Read the model definition and answer for the solid it produces. Units are mm, in the model's axes. A direction names the side the tool comes from. Round coordinates to 2 decimals unless told otherwise and drop trailing zeros. Write each loop counter-clockwise with the first axis right and the second up, starting at its lowest first coordinate (ties: lowest second). Pieces come first, ordered by that corner, then holes.
from build123d import *

# Parameters (mm, degrees)
F0_W     = 145
F0_H     = 185
F1_DEPTH = 55
F3_DEPTH = 98
F5_W     = 120
F5_H     = 28
F6_DEPTH = 25
F7_R     = 5


with BuildPart() as f1:
    # F0 (on Top) → F1 (new body)
    with BuildSketch(Plane.XY):
        Rectangle(F0_W, F0_H)
    extrude(amount=F1_DEPTH)

    # F2 (on Front) → F3 (cut, symmetric)
    with BuildSketch(Plane.XZ):
        Polygon((-92.57464, 55.003494), (-92.79651, 32.817475), (26.113287, 32.817475), (47.771066, 55.003494), align=None)
    extrude(amount=F3_DEPTH, both=True, mode=Mode.SUBTRACT)

    # F5 (on face) → F6 (cut)
    with BuildSketch(Plane.YZ.offset(72.5)):
        with Locations((0.170817, 26)):
            Rectangle(F5_W, F5_H)
    extrude(amount=-F6_DEPTH, mode=Mode.SUBTRACT)

    # F7
    f7_edges = [f1.edges().sort_by_distance(p)[0] for p in [
        (-23.193357, -92.5, 32.817475),
        (36.940471, -92.5, 43.908738),
        (-72.5, 0, 32.817475),
        (-23.193357, 92.5, 32.817475),
        (36.940471, 92.5, 43.908738),
        (47.767656, 0, 55),
        (72.5, 0, 55),
        (60.133828, -92.5, 55),
        (72.5, -92.5, 27.5),
        (72.5, 92.5, 27.5),
        (60.133828, 92.5, 55),
        (0, -92.5, 0),
        (0, 92.5, 0),
        (-72.5, 0, 0),
        (-72.5, -92.5, 16.408738),
        (-72.5, 92.5, 16.408738),
    ]]
    fillet(f7_edges, radius=F7_R)


solid = f1.part
Q1. Section C-C (z = 18) is taken. Determine the outline of the cut face in (x, y), then the cut area to 3 significant figures.
Verdict:
outline: (-72.5, -87.5) arc R5 ccw to (-67.5, -92.5) - (67.5, -92.5) arc R5 ccw to (72.5, -87.5) - (72.5, -59.83) - (47.5, -59.83) - (47.5, 60.17) - (72.5, 60.17) - (72.5, 87.5) arc R5 ccw to (67.5, 92.5) - (-67.5, 92.5) arc R5 ccw to (-72.5, 87.5) - close
area: 23,800 mm2
Q2. Which of the six approach directions +Z, -Z, +X, -X, +Y, -Y give full straight-line access (tool end or side, diameter ignored) to faces 5 (the cylindrical face through (-20.31, -91, 31.39)), 6 (the cylindrical face through (-20.31, 91.074, 31.314)), 7 (the flat face through (60, -1, 40))?
Verdict:
face 5: +Z, -X, -Y
face 6: +Z, -X, +Y
face 7: +X
Q3. Flat-ended cylindrical pins translate along their axes: pin 1 Ø3 at (x, y) = (-46.5, -45) entering from +Z; pin 2 Ø3 at (y, z) = (-39, 49) entering from -X; pin 3 Ø8.5 at (y, z) = (-8.5, 28.5) entering from +X. Find the tip coordinate at first contact, or state that the pin passes through.
Verdict:
pin 1: stops at z = 32.82
pin 2: stops at x = 40.45
pin 3: stops at x = 47.5
Q4. Section A-A (y = 56) is taken. Determine the outline of the cut face in (x, z), then the cut area to 3 significant figures.
Verdict:
outline: (-72.5, 5) arc R5 ccw to (-67.5, 0) - (72.5, 0) - (72.5, 12) - (47.5, 12) - (47.5, 40) - (72.5, 40) - (72.5, 50) arc R5 ccw to (67.5, 55) - (49.87, 55) arc R5 ccw to (46.3, 53.49) - (26.11, 32.82) - (-67.5, 32.82) arc R5 ccw to (-72.5, 27.82) - close
area: 4,830 mm2
Q5. Straight lines are drawn through the part: probe 1 along Y at (x, z) = (54.5, 35.5); probe 2 along Z at (x, y) = (51, 55); probe 3 along Z at (x, y) = (7, -3). For each, find the intervals that lie inside material, in ascending order.
Verdict:
probe 1: y = -92.5 to -59.83, 60.17 to 92.5
probe 2: z = 0 to 12, 40 to 55
probe 3: z = 0 to 32.82
Q6. Section D-D (y = 77.5) is taken. Determine the outline of the cut face in (x, z), then the cut area to 3 significant figures.
Verdict:
outline: (-72.5, 5) arc R5 ccw to (-67.5, 0) - (72.5, 0) - (72.5, 50) arc R5 ccw to (67.5, 55) - (49.87, 55) arc R5 ccw to (46.3, 53.49) - (26.11, 32.82) - (-67.5, 32.82) arc R5 ccw to (-72.5, 27.82) - close
area: 5,530 mm2
Q7. Section B-B (x = -36.5) is taken. Determine the outline of the cut face in (y, z), then the cut area to 3 significant figures.
Verdict:
outline: (-92.5, 5) arc R5 ccw to (-87.5, 0) - (87.5, 0) arc R5 ccw to (92.5, 5) - (92.5, 27.82) arc R5 ccw to (87.5, 32.82) - (-87.5, 32.82) arc R5 ccw to (-92.5, 27.82) - close
area: 6,050 mm2
Q8. Determine the mould class of faces 1 (the cylindrical face through (3.48, -91, 1.43)), 2 (the flat face through (72.5, -1, 41)), 3 (the flat face through (47.5, -1, 26)), 4 (the cylindrical face through (36.39, 91.07, 41.2)) for opening direction Y: pulls with the +Y half, pulls with the -Y half, needs draft (parallel to the pull), parting line crosses it, or undercut.
Verdict:
face 1: pulls with the -Y half
face 2: needs draft
face 3: undercut
face 4: pulls with the +Y half
